Part model, mm, in its own coordinate system. A direction names the side the tool comes from. Give positions to 0.01 mm unless a question says otherwise; leave off trailing zeros. Order: outer loops, then holes, each group sorted by start corner. A loop starts at its lowest first (then second) coordinate and runs counter-clockwise, first axis right, second up.
1. Mould opens along X. For faces 1 (the flat face through (-2.2, 3.175, -530.7)), 2 (the flat face through (-2, 0, -530)), 3 (the flat face through (3.175, 0, -531)), 4 (the flat face through (-3.175, 0, -531)) say: +X half, -X half, draft (parallel to the pull), parting line (faces both ways), or undercut.
2. Probe line 1 (Z direction, x = 0.5, y = 0); line 2 (Z direction, x = 1.5, y = -3); line 3 (Y direction, x = 2.25, z = -599.6) (3 decimals). List the from-to ranges inside material, lowest first.
3. Drop a flat-ended pin along its axis: pin 1 Ø2 at (y, z) = (0, -599.6) entering from +X. Give the stop position or say it passes through.
4. Slice it at C-C on x = 0. List the corners of the cut face in (y, z) (3 decimals), and give its area (3 significant figures).
5. Which spindle directions (+Z, -Z, +X, -X, +Y, -Y) get a long thin tool onto all of the face, cutting with end or side? Do faces 5 (the cylindrical face through (0.044, -0.67, -457.983)), 6 (the flat face through (0, 0, -531.6)). Say none if no direction does.
6. Slice it at A-A on y = 0. List the corners of the cut face in (x, z) (3 decimals).
7. Slice it at B-B on z = -599.6. List the corners of the cut face in (x, y) (3 decimals).
from build123d import *

# Parameters (mm, degrees)
BOSS_EXTRUDE1_DEPTH      = 609.6
BOSS_EXTRUDE1_DEPTH_BACK = 609.6
SKETCH3_W                = 6.35
SKETCH3_H                = 6.35
SKETCH4_W                = 7.35
SKETCH4_H                = 7.35
CUT_EXTRUDE1_DEPTH       = 1060.209517164
SKETCH5_R                = 1.75
CUT_EXTRUDE2_DEPTH       = 610.641339744
SKETCH6_W                = 4
SKETCH6_H                = 4
CUT_EXTRUDE3_DEPTH       = 610.641339744


with BuildPart() as part:
    # Sketch3 → Boss-Extrude1 (new, two sides: drawn at the far end of the back side and taken through both)
    with BuildSketch(Plane.XY.offset(-BOSS_EXTRUDE1_DEPTH_BACK)):
        Rectangle(SKETCH3_W, SKETCH3_H)
    extrude(amount=BOSS_EXTRUDE1_DEPTH + BOSS_EXTRUDE1_DEPTH_BACK)

    # Sketch4 → Cut-Extrude1 (cut, through all)
    with BuildSketch(Plane(origin=(0, 0, -449.6), x_dir=(-1, 0, 0), z_dir=(0, 0, -1))):
        Rectangle(SKETCH4_W, SKETCH4_H)
    extrude(amount=-CUT_EXTRUDE1_DEPTH, mode=Mode.SUBTRACT)

    # Sketch5 → Cut-Extrude2 (cut, through all)
    with BuildSketch(Plane(origin=(3.175, 0, 0), x_dir=(0, 1, 0), z_dir=(-1, 0, 0))):
        with Locations(Location((0, 599.6, 0), (0, 0, 270))):
            Circle(SKETCH5_R)
        with Locations(Location((0, 459.6, 0), (0, 0, 270))):
            Circle(SKETCH5_R)
    extrude(amount=CUT_EXTRUDE2_DEPTH, mode=Mode.SUBTRACT)

    # Sketch6 → Cut-Extrude3 (cut, through all)
    with BuildSketch(Plane(origin=(0, 3.175, 0), x_dir=(1, 0, 0), z_dir=(0, 1, 0))):
        with Locations((0, 529.6)):
            Rectangle(SKETCH6_W, SKETCH6_H)
    extrude(amount=-CUT_EXTRUDE3_DEPTH, mode=Mode.SUBTRACT)


solid = part.part
Data:
1. face 1: draft
1. face 2: undercut
1. face 3: +X half
1. face 4: -X half
2. line 1: z = -609.6 to -601.35, -597.85 to -531.6, -527.6 to -461.35, -457.85 to -449.6
2. line 2: z = -609.6 to -531.6, -527.6 to -449.6
2. line 3: y = -3.175 to -1.75, 1.75 to 3.175
3. pin 1: passes through
4. outline: (-3.175, -609.6) - (3.175, -609.6) - (3.175, -531.6) - (-3.175, -531.6) - close; (-3.175, -527.6) - (3.175, -527.6) - (3.175, -449.6) - (-3.175, -449.6) - close; hole circle Ø3.5 at (0, -599.6); hole circle Ø3.5 at (0, -459.6)
4. area: 971 mm2
5. face 5: +X, -X
5. face 6: +Y, -Y
6. outline: (-3.175, -609.6) - (3.175, -609.6) - (3.175, -601.35) - (-3.175, -601.35) - close; (-3.175, -597.85) - (3.175, -597.85) - (3.175, -461.35) - (-3.175, -461.35) - close; (-3.175, -457.85) - (3.175, -457.85) - (3.175, -449.6) - (-3.175, -449.6) - close; hole (-2, -531.6) - (2, -531.6) - (2, -527.6) - (-2, -527.6) - close
7. outline: (-3.175, -3.175) - (3.175, -3.175) - (3.175, -1.75) - (-3.175, -1.75) - close; (-3.175, 1.75) - (3.175, 1.75) - (3.175, 3.175) - (-3.175, 3.175) - close
